from build123d import *

# Parameters (mm, degrees)
SKICA1_R                      = 45
P_IDAT_VYSUNUT_M1_DEPTH       = 12
SKICA2_R                      = 25
P_IDAT_VYSUNUT_M2_DEPTH       = 30
P_IDAT_VYSUNUT_M2_TAPER       = 3
ODEBRAT_VYSUNUT_M1_REACH      = 78.25
SKICA3_R                      = 15
ODEBRAT_VYSUNUT_M2_REACH      = 78.25
SKICA4_W                      = 10
SKICA4_H                      = 3.370987204
ZAOBLIT1_R                    = 2
ODEBRAT_VYSUNUT_M3_REACH      = 72.356
SKICA5_R                      = 4.5
ZKOSEN_1_SIZE                 = 0.5
KRUHOV_POLE1_COUNT            = 6
ZKOSEN_1_OF_KRUHOV_POLE1_SIZE = 0.5
ZAOBLIT2_R                    = 0.5
ZKOSEN_2_SIZE                 = 1.056754503
ZKOSEN_2_SIZE_2               = 1


with BuildPart() as part:
    # Skica1 → Přidat vysunutím1 (new body)
    with BuildSketch(Plane.XY):
        Circle(SKICA1_R)
    extrude(amount=P_IDAT_VYSUNUT_M1_DEPTH)

    # Skica2 → Přidat vysunutím2 (add)
    with BuildSketch(Plane.XY.offset(12)):
        Circle(SKICA2_R)
    extrude(amount=P_IDAT_VYSUNUT_M2_DEPTH, taper=P_IDAT_VYSUNUT_M2_TAPER)

    # Skica3 → Odebrat vysunutím1 (cut, up to next)
    with BuildSketch(Plane.XY.offset(42), mode=Mode.PRIVATE) as odebrat_vysunut_m1_sk1:
        Circle(SKICA3_R)
    odebrat_vysunut_m1_tool1 = extrude(odebrat_vysunut_m1_sk1.sketch, amount=-ODEBRAT_VYSUNUT_M1_REACH, mode=Mode.PRIVATE) & part.part
    add(odebrat_vysunut_m1_tool1.solids().sort_by_distance((0, 0, 42))[0], mode=Mode.SUBTRACT)

    # Skica4 → Odebrat vysunutím2 (cut, up to next)
    with BuildSketch(Plane.XY.offset(42), mode=Mode.PRIVATE) as odebrat_vysunut_m2_sk1:
        with Locations((0, 14.814506398)):
            Rectangle(SKICA4_W, SKICA4_H)
    odebrat_vysunut_m2_tool1 = extrude(odebrat_vysunut_m2_sk1.sketch, amount=-ODEBRAT_VYSUNUT_M2_REACH, mode=Mode.PRIVATE) & part.part
    add(odebrat_vysunut_m2_tool1.solids().sort_by_distance((0, 14.814506, 42))[0], mode=Mode.SUBTRACT)

    # Zaoblit1
    zaoblit1_edges = [part.edges().sort_by_distance(p)[0] for p in [
        (-25, 0, 12),
    ]]
    fillet(zaoblit1_edges, radius=ZAOBLIT1_R)

    # Skica5 → Odebrat vysunutím3 (cut, up to next)
    with BuildSketch(Plane.XY.offset(12), mode=Mode.PRIVATE) as odebrat_vysunut_m3_sk1:
        with Locations((35, 0)):
            Circle(SKICA5_R)
    odebrat_vysunut_m3_tool1 = extrude(odebrat_vysunut_m3_sk1.sketch, amount=-ODEBRAT_VYSUNUT_M3_REACH, mode=Mode.PRIVATE) & part.part
    odebrat_vysunut_m3 = odebrat_vysunut_m3_tool1.solids().sort_by_distance((35, 0, 12))[0]
    add(odebrat_vysunut_m3, mode=Mode.SUBTRACT)

    # Zkosení1
    zkosen_1_edges = [part.edges().sort_by_distance(p)[0] for p in [
        (30.5, 0, 12),
    ]]
    chamfer(zkosen_1_edges, length=ZKOSEN_1_SIZE)

    # Kruhové pole1: Odebrat vysunutím3 ×6 about axis
    kruhov_pole1_axis = Axis((0, 0, 0), (0, 0, 1))
    for i in range(1, KRUHOV_POLE1_COUNT):
        add(odebrat_vysunut_m3.rotate(kruhov_pole1_axis, i * 360 / KRUHOV_POLE1_COUNT), mode=Mode.SUBTRACT)

    # Zkosení1 of Kruhové pole1
    zkosen_1_of_kruhov_pole1_edges = [part.edges().sort_by_distance(p)[0] for p in [
        (15.25, 26.413774815, 12),
        (-15.25, 26.413774815, 12),
        (-30.5, 0, 12),
        (-15.25, -26.413774815, 12),
        (15.25, -26.413774815, 12),
    ]]
    chamfer(zkosen_1_of_kruhov_pole1_edges, length=ZKOSEN_1_OF_KRUHOV_POLE1_SIZE)

    # Zaoblit2
    zaoblit2_edges = [part.edges().sort_by_distance(p)[0] for p in [
        (-5, 16.5, 21),
        (5, 16.5, 21),
    ]]
    fillet(zaoblit2_edges, radius=ZAOBLIT2_R)

    # Zkosení2
    # the kernel refuses this chamfer: 1.056754503, 1 mm, written as the material it takes off along each edge
    with BuildSketch(Plane(origin=(0, 0, 42), x_dir=(1, 0, 0), z_dir=(0, 1, 0))) as zkosen_2_piece_1:
        Polygon((23.427766622 - ZKOSEN_2_SIZE, 0), (23.427766622 + ZKOSEN_2_SIZE_2 * 0.0523359562429, ZKOSEN_2_SIZE_2 * 0.998629534755), (23.427766622, 0), align=None)
    revolve(axis=Axis((0, 0, 42), (0, 0, -1)), mode=Mode.SUBTRACT)


solid = part.part
Verification items for the finished model (mm, model axes). A direction names the side the tool comes from. Coordinates: 2 decimals unless noted, no trailing zeros. Loops run counter-clockwise (first coordinate to the right, second up) from the corner with the lowest first, then second, coordinate; pieces in that order, holes last. Notation, with made-up numbers: (-21.75, 61) -> (3.25, 61) arc R18 ccw to (3.25, 69) -> close; hole circle Ø6 at (-11.75, 41). An arc over 180 degrees is marked (long way). Answer as a JSON object with one key per item and string values. Group by question number.
Item 1: Scan lines: probe 1 along X at (y, z) = (31.5, 11); probe 2 along Y at (x, z) = (17.5, 8.75); probe 3 along Y at (x, z) = (-17, 8). Record each from-to range of solid material in increasing order.
Item 2: Depth check by flat-ended pin: pin 1 (10 mm diameter, centred on x = -24, z = 32.5, fed in from -Y); pin 2 (10 mm diameter, centred on x = -1, z = 30.5, fed in from +Y); pin 3 (6 mm diameter, centred on x = 24, z = 37.5, fed in from +Y). Enter the tip coordinate at first touch or a pass-through.
Item 3: Sectioned sample at C-C on z = 6.5. Record the boundary of the cut face in (x, y).
Item 4: Tool access check on faces 1 (the flat face through (5, -15, 42)), 2 (the flat face through (0, 16.5, 21)). Record the directions out of +Z, -Z, +X, -X, +Y, -Y that give a thin tool (end or side, any length) a straight path to the whole face; none if there is none.
Item 5: Sectioned sample at D-D on z = 30. Record the boundary of the cut face in (x, y).
Item 6: Mould release check, pull along Y, two halves, no side actions. Record for faces 3 (the cylindrical face through (-15.42, 26.32, 5.83)), 4 (the conical face through (-5.242, -23.605, 27.638)), 5 (the flat face through (19.4, -19.4, 12)): +Y half, -Y half, draft (parallel to the pull), parting line (faces both ways), or undercut.
Item 7: Sectioned sample at B-B on x = 0. Record the boundary of the cut face in (y, z).
Item 8: Sectioned sample at A-A on y = 0. Record the boundary of the cut face in (x, z).
Evaluation:
{
 "1": {"probe 1": "x = -32.14 to -21.84, -13.16 to 13.16, 21.84 to 32.14", "probe 2": "y = -41.46 to -34.81, -25.81 to 25.81, 34.81 to 41.46", "probe 3": "y = -41.67 to -34.78, -25.84 to 25.84, 34.78 to 41.67"},
 "2": {"pin 1": "stops at y = -14.56", "pin 2": "stops at y = 24.29", "pin 3": "stops at y = 10.92"},
 "3": {"outline": "circle Ø90 at (0, 0); hole circle Ø9 at (-35, 0); hole circle Ø9 at (-17.5, -30.31); hole circle Ø9 at (-17.5, 30.31); hole (-5, 14.14) arc R15 ccw (long way) to (5, 14.14) -> (5, 16) arc R0.5 ccw to (4.5, 16.5) -> (-4.5, 16.5) arc R0.5 ccw to (-5, 16) -> close; hole circle Ø9 at (17.5, -30.31); hole circle Ø9 at (17.5, 30.31); hole circle Ø9 at (35, 0)"},
 "4": {"face 1": "+Z, +X, -X, +Y, -Y", "face 2": "+Z, -Z"},
 "5": {"outline": "circle Ø48.11 at (0, 0); hole (-5, 14.14) arc R15 ccw (long way) to (5, 14.14) -> (5, 16) arc R0.5 ccw to (4.5, 16.5) -> (-4.5, 16.5) arc R0.5 ccw to (-5, 16) -> close"},
 "6": {"face 3": "undercut", "face 4": "parting line", "face 5": "draft"},
 "7": {"outline": "(-45, 0) -> (-15, 0) -> (-15, 42) -> (-22.37, 42) -> (-23.48, 41) -> (-24.9, 13.9) arc R2 cw to (-26.9, 12) -> (-45, 12) -> close; (16.5, 0) -> (45, 0) -> (45, 12) -> (26.9, 12) arc R2 cw to (24.9, 13.9) -> (23.48, 41) -> (22.37, 42) -> (16.5, 42) -> close"},
 "8": {"outline": "(-45, 0) -> (-39.5, 0) -> (-39.5, 11.5) -> (-40, 12) -> (-45, 12) -> close; (-30.5, 0) -> (-15, 0) -> (-15, 42) -> (-22.37, 42) -> (-23.48, 41) -> (-24.9, 13.9) arc R2 cw to (-26.9, 12) -> (-30, 12) -> (-30.5, 11.5) -> close; (15, 0) -> (30.5, 0) -> (30.5, 11.5) -> (30, 12) -> (26.9, 12) arc R2 cw to (24.9, 13.9) -> (23.48, 41) -> (22.37, 42) -> (15, 42) -> close; (39.5, 0) -> (45, 0) -> (45, 12) -> (40, 12) -> (39.5, 11.5) -> close"}
}
